Geometry check sheet. Reference: the model listing, model coordinates, mm. Face numbers are marked on the shaded views. A direction names the side the tool comes from. Give positions to 0.01 mm unless a question says otherwise; leave off trailing zeros. Loops run counter-clockwise (first coordinate to the right, second up) from the corner with the lowest first, then second, coordinate; pieces in that order, holes last. Notation, with made-up numbers: (85, 5) -> (129, 5) arc R22 cw to (129, 35) -> close; hole circle Ø7 at (38, 74). An arc over 180 degrees is marked (long way). Answer as a JSON object with one key per item and string values.
from build123d import *

# Parameters (mm, degrees)
EXTRUDE_1_DEPTH          = 300
SHELL_1_T                = -2
SKETCH_3_W               = 101.211387706
SKETCH_3_H               = 60
CUT_EXTRUDE_1_DEPTH      = 296
EXTRUDE_2_DEPTH          = 300
CUT_EXTRUDE_2_DEPTH      = 541.092584656
CUT_EXTRUDE_2_DEPTH_BACK = 541.092584656
SKETCH_6_R               = 4


with BuildPart() as part:
    # 草图1 → 凸台-拉伸1 (new body)
    with BuildSketch(Plane.XY):
        with BuildLine():
            Line((-22.839294621, -20), (-87.749643874, -20))
            ThreePointArc((-87.749643874, -20), (-56.124860802, -70.356236397), (0, -90))
            Line((0, -90), (400, -90))
            Line((400, -90), (426.457513111, -90))
            ThreePointArc((426.457513111, -90), (436.457513111, -76.457513111), (440, -60))
            Line((440, -60), (440, -20))
            Line((440, -20), (400, -20))
            Line((400, -20), (-22.839294621, -20))
        make_face()
    extrude(amount=-EXTRUDE_1_DEPTH)

    # 抽壳1
    shell_1_openings = [part.faces().sort_by_distance(p)[0] for p in [
        (176.125178063, -20, -150),
    ]]
    offset(amount=SHELL_1_T, openings=shell_1_openings, kind=Kind.INTERSECTION)

    # 草图3 → 切除-拉伸1 (cut)
    with BuildSketch(Plane.XY.offset(-298)):
        with Locations((-50.605693853, -60)):
            Rectangle(SKETCH_3_W, SKETCH_3_H)
    extrude(amount=CUT_EXTRUDE_1_DEPTH, mode=Mode.SUBTRACT)

    # 草图4 → 凸台-拉伸2 (add)
    with BuildSketch(Plane.XY):
        with BuildLine():
            Line((85.697141143, -20), (87.749643874, -20))
            ThreePointArc((87.749643874, -20), (56.124860802, -70.356236397), (0, -90))
            Line((0, -90), (0, -88))
            ThreePointArc((0, -88), (54.699177325, -68.934751758), (85.697141143, -20))
        make_face()
    extrude(amount=-EXTRUDE_2_DEPTH)

    # 草图6 → 切除-拉伸2 (cut, two sides: drawn at the far end of the back side and taken through both)
    with BuildSketch(Plane.XY.offset(-CUT_EXTRUDE_2_DEPTH_BACK)):
        with Locations((400, -60)):
            Circle(SKETCH_6_R)
    extrude(amount=CUT_EXTRUDE_2_DEPTH + CUT_EXTRUDE_2_DEPTH_BACK, mode=Mode.SUBTRACT)


solid = part.part
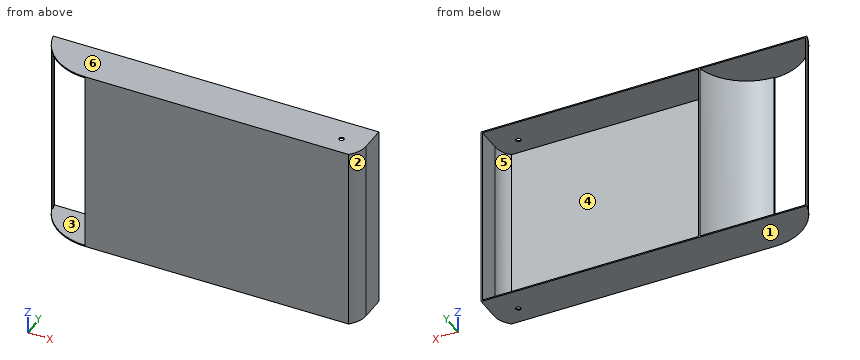
1) Section check A-A on z = -114.5. Record the cut outline in (x, y), plus the area to 3 significant figures.
Geometry check:
{"outline": "(-87.75, -20) arc R90 ccw to (-84.85, -30) -> (-82.73, -30) arc R88 cw to (-85.7, -20) -> close; (0, -90) -> (426.46, -90) arc R40 ccw to (440, -60) -> (440, -20) -> (438, -20) -> (438, -60) arc R38 cw to (425.69, -88) -> (18.87, -88) arc R90 ccw to (87.75, -20) -> (85.7, -20) arc R88 cw to (0, -88) -> close", "area": "1,230 mm2"}
2) Section check D-D on x = 139. Record the cut outline in (y, z).
Geometry check:
{"outline": "(-90, -300) -> (-20, -300) -> (-20, -298) -> (-88, -298) -> (-88, -2) -> (-20, -2) -> (-20, 0) -> (-90, 0) -> close"}
3) Section check C-C on x = 46. Record the cut outline in (y, z).
Geometry check:
{"outline": "(-90, -300) -> (-20, -300) -> (-20, -298) -> (-75.02, -298) -> (-75.02, -2) -> (-20, -2) -> (-20, 0) -> (-90, 0) -> close; hole (-88, -298) -> (-77.36, -298) -> (-77.36, -2) -> (-88, -2) -> close"}
4) Material ranges on line 1 along Z through (x, y) = (72.5, -25); line 2 along Y through (x, z) = (400, -299); line 3 along Y through (x, z) = (129.5, -87), recorded low to high. Write a range as from..to.
Geometry check:
{"line 1": "z = -300..-298, -2..0", "line 2": "y = -90..-64, -56..-20", "line 3": "y = -90..-88"}
5) Depth check by flat-ended pin: P1, Ø5, axis at x = 400, y = -60, coming from the -Z side; P2, Ø1.5, axis at y = -80.5, z = -174.5, coming from the +X side; P3, Ø2.5, axis at x = -84, z = -77.5, coming from the -Y side; P4, Ø2, axis at y = -89.5, z = -139, coming from the -X side. Enter the tip coordinate at first touch or a pass-through.
Geometry check:
{"P1": "passes through", "P2": "stops at x = 434.78", "P3": "stops at y = -30", "P4": "stops at x = 0"}
6) Tool access check on the marked faces 4, 5 and 6. Record the directions out of +Z, -Z, +X, -X, +Y, -Y that give a thin tool (end or side, any length) a straight path to the whole face; none if there is none.
Geometry check:
{"face 4": "none", "face 5": "+Y", "face 6": "+Z, +X, -X, +Y, -Y"}
7) Draft check along X on the marked faces 1, 2 and 3. Enter one of: pulls with the +X half, pulls with the -X half, needs draft (parallel to the pull), parting line crosses it, or undercut.
Geometry check:
{"face 1": "needs draft", "face 2": "pulls with the +X half", "face 3": "undercut"}
8) Section check B-B on y = -69. Record the cut outline in (x, z), plus the area to 3 significant figures.
Geometry check:
{"outline": "(-57.78, -300) -> (438.97, -300) -> (438.97, 0) -> (-57.78, 0) -> (-57.78, -2) -> (54.62, -2) -> (54.62, -298) -> (-57.78, -298) -> close; hole (57.78, -298) -> (436.92, -298) -> (436.92, -2) -> (57.78, -2) -> close", "area": "3,530 mm2"}
